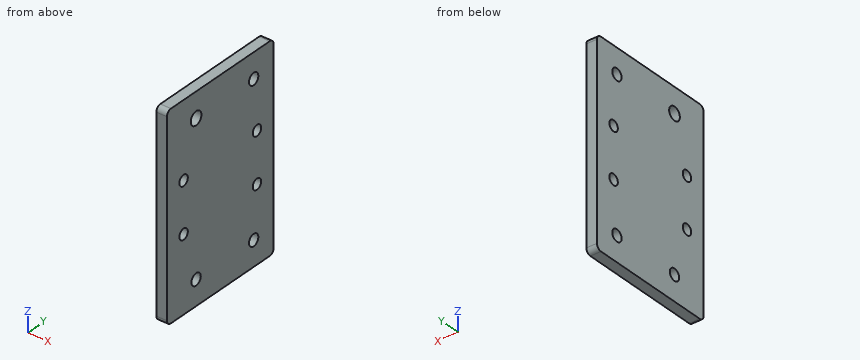
```python
from build123d import *

# Parameters (mm, degrees)
SKETCH1_W           = 120
SKETCH1_H           = 80
SKETCH1_R           = 3.5
SKETCH1_R_2         = 4
BOSS_EXTRUDE1_DEPTH = 6.35
FILLET1_R           = 3
SKETCH2_R           = 3.175
CUT_EXTRUDE1_DEPTH  = 10


with BuildPart() as part:
    # Sketch1 → Boss-Extrude1 (new body)
    with BuildSketch(Plane(origin=(0, 0, 0), x_dir=(0, 0, -1), z_dir=(1, 0, 0))):
        Rectangle(SKETCH1_W, SKETCH1_H)
        with Locations((45, 25)):
            Circle(SKETCH1_R, mode=Mode.SUBTRACT)
        with Locations((-45, 25)):
            Circle(SKETCH1_R, mode=Mode.SUBTRACT)
        with Locations((-45, -18.13)):
            Circle(SKETCH1_R_2, mode=Mode.SUBTRACT)
        with Locations((45, -18.13)):
            Circle(SKETCH1_R, mode=Mode.SUBTRACT)
    extrude(amount=BOSS_EXTRUDE1_DEPTH)

    # Fillet1
    fillet1_edges = [part.edges().sort_by_distance(p)[0] for p in [
        (3.175, -40, -60),
        (3.175, -40, 60),
        (3.175, 40, 60),
        (3.175, 40, -60),
    ]]
    fillet(fillet1_edges, radius=FILLET1_R)

    # Sketch2 → Cut-Extrude1 (cut)
    with BuildSketch(Plane(origin=(6.35, 0, 0), x_dir=(0, 0, -1), z_dir=(1, 0, 0))):
        with Locations((-15, 27.5)):
            Circle(SKETCH2_R)
        with Locations((15, 27.5)):
            Circle(SKETCH2_R)
        with Locations((15, -27.5)):
            Circle(SKETCH2_R)
        with Locations((-15, -27.5)):
            Circle(SKETCH2_R)
    extrude(amount=-CUT_EXTRUDE1_DEPTH, mode=Mode.SUBTRACT)


solid = part.part
```
Verification items for the finished model (mm, model axes). Round coordinates to 2 decimals unless told otherwise and drop trailing zeros. Write each loop counter-clockwise with the first axis right and the second up, starting at its lowest first coordinate (ties: lowest second). Pieces come first, ordered by that corner, then holes. Notation, with made-up numbers: (45.25, 83.25) -> (91.25, 83.25) arc R22 ccw to (91.25, 109.25) -> close; hole circle Ø9 at (14.25, -2). An arc over 180 degrees is marked (long way). Write each question's results on one line, items separated by ' | '.
Q1. Go/stop test with a flat-tipped pin: pin 1 Ø5.5 at (y, z) = (27.5, -15) entering from +X. Record where the tip stops, or that it passes through.
Derived:
pin 1: passes through
Q2. Sectioned sample at C-C, the plane x = 4.5. Give the number of separate pieces and of enclosed holes in the cut face, and give its area (3 significant figures).
Derived:
separate pieces: 1 | enclosed holes: 8 | area: 9,300 mm²
Q3. Thickness scan on probe 1 along Y at (x, z) = (2, -15) (3 decimals); probe 2 along Y at (x, z) = (3, -45); probe 3 along Z at (x, y) = (2, 22). Record the ranges inside material, lowest first.
Derived:
probe 1: y = -40 to -30.675, -24.325 to 24.325, 30.675 to 40 | probe 2: y = -40 to -21.63, -14.63 to 21.5, 28.5 to 40 | probe 3: z = -60 to -46.8, -43.2 to 43.2, 46.8 to 60
Q4. Sectioned sample at A-A, the plane z = 15. Record the boundary of the cut face in (x, y) (3 decimals).
Derived:
outline: (0, -40) -> (6.35, -40) -> (6.35, -30.675) -> (0, -30.675) -> close; (0, -24.325) -> (6.35, -24.325) -> (6.35, 24.325) -> (0, 24.325) -> close; (0, 30.675) -> (6.35, 30.675) -> (6.35, 40) -> (0, 40) -> close
Q5. Sectioned sample at B-B, the plane y = -18.13. Record the boundary of the cut face in (x, z), and give its area (3 significant figures).
Derived:
outline: (0, -60) -> (6.35, -60) -> (6.35, -48.5) -> (0, -48.5) -> close; (0, -41.5) -> (6.35, -41.5) -> (6.35, 41) -> (0, 41) -> close; (0, 49) -> (6.35, 49) -> (6.35, 60) -> (0, 60) -> close | area: 667 mm²
